from build123d import *

# Parameters (mm, degrees)
SKETCH4_R          = 3
CUT_EXTRUDE1_DEPTH = 1
CUT_EXTRUDE2_START = -3
SKETCH5_R          = 3
CUT_EXTRUDE2_DEPTH = 3
CUT_EXTRUDE3_REACH = 19.282
SKETCH6_R          = 1.143
SKETCH6_R_2        = 1.1938


with BuildPart() as part:
    # Sketch1 → Revolve1 (revolve)
    with BuildSketch(Plane.XY, mode=Mode.PRIVATE) as revolve1_sk:
        Polygon((-12, 0), (-3.75, 0), (-3.75, 1.732400048), (-1.4, 1.732400048), (-1.4, -3.267599952), (-4.45, -3.267599952), (-4.45, -1.700599952), (-12, -1.700599952), align=None)
    revolve(revolve1_sk.sketch.rotate(Axis((0, 0, 0), (0, -1, 0)), 270), axis=Axis((0, 0, 0), (0, -1, 0)))

    # Sketch4 → Cut-Extrude1 (cut)
    with BuildSketch(Plane(origin=(0, 1.732400048, 0), x_dir=(-1, 0, 0), z_dir=(0, 1, 0))):
        with Locations(Location((0, 0, 0), (0, 0, 90))):
            Circle(SKETCH4_R)
    extrude(amount=-CUT_EXTRUDE1_DEPTH, mode=Mode.SUBTRACT)

    # Sketch5 → Cut-Extrude2 (cut)
    with BuildSketch(Plane.XZ.offset(3.267599952).offset(CUT_EXTRUDE2_START)):
        with Locations(Location((0, 0, 0), (0, 0, 90))):
            Circle(SKETCH5_R)
    extrude(amount=CUT_EXTRUDE2_DEPTH, mode=Mode.SUBTRACT)

    # Sketch6 → Cut-Extrude3 (cut, up to next)
    with BuildSketch(Plane(origin=(0, 0, 0), x_dir=(1, 0, 0), z_dir=(0, 1, 0)), mode=Mode.PRIVATE) as cut_extrude3_sk1:
        with Locations(Location((0, 8.3312, 0), (0, 0, 270))):
            Circle(SKETCH6_R)
    cut_extrude3_tool1 = extrude(cut_extrude3_sk1.sketch, amount=-CUT_EXTRUDE3_REACH, mode=Mode.PRIVATE) & part.part
    # Sketch6 → Cut-Extrude3 (cut, up to next)
    with BuildSketch(Plane(origin=(0, 0, 0), x_dir=(1, 0, 0), z_dir=(0, 1, 0)), mode=Mode.PRIVATE) as cut_extrude3_sk2:
        with Locations(Location((-8.3312, 0, 0), (0, 0, 270))):
            Circle(SKETCH6_R)
    cut_extrude3_tool2 = extrude(cut_extrude3_sk2.sketch, amount=-CUT_EXTRUDE3_REACH, mode=Mode.PRIVATE) & part.part
    # Sketch6 → Cut-Extrude3 (cut, up to next)
    with BuildSketch(Plane(origin=(0, 0, 0), x_dir=(1, 0, 0), z_dir=(0, 1, 0)), mode=Mode.PRIVATE) as cut_extrude3_sk3:
        with Locations(Location((0, -8.3312, 0), (0, 0, 270))):
            Circle(SKETCH6_R)
    cut_extrude3_tool3 = extrude(cut_extrude3_sk3.sketch, amount=-CUT_EXTRUDE3_REACH, mode=Mode.PRIVATE) & part.part
    # Sketch6 → Cut-Extrude3 (cut, up to next)
    with BuildSketch(Plane(origin=(0, 0, 0), x_dir=(1, 0, 0), z_dir=(0, 1, 0)), mode=Mode.PRIVATE) as cut_extrude3_sk4:
        with Locations(Location((8.3312, 0, 0), (0, 0, 270))):
            Circle(SKETCH6_R_2)
    cut_extrude3_tool4 = extrude(cut_extrude3_sk4.sketch, amount=-CUT_EXTRUDE3_REACH, mode=Mode.PRIVATE) & part.part
    add(cut_extrude3_tool1.solids().sort_by_distance((0, 0, -8.3312))[0], mode=Mode.SUBTRACT)
    add(cut_extrude3_tool2.solids().sort_by_distance((-8.3312, 0, 0))[0], mode=Mode.SUBTRACT)
    add(cut_extrude3_tool3.solids().sort_by_distance((0, 0, 8.3312))[0], mode=Mode.SUBTRACT)
    add(cut_extrude3_tool4.solids().sort_by_distance((8.3312, 0, 0))[0], mode=Mode.SUBTRACT)


solid = part.part
Build history of the part. All positions in model axes, mm. A direction names the side the tool comes from. Round coordinates to 2 decimals unless told otherwise and drop trailing zeros. Loops run counter-clockwise (first coordinate to the right, second up) from the corner with the lowest first, then second, coordinate; pieces in that order, holes last. Notation, with made-up numbers: (-28.75, 77.25) -> (3.25, 77.25) arc R29 cw to (3.25, 102.25) -> close; hole circle Ø1 at (-17, 40.5). An arc over 180 degrees is marked (long way). One line per item, written item: value. Start each with the question number.
Q1. Cut at C-C on y = 1.05. List the corners of the cut face in (x, z), plus the area to 3 significant figures.
Q2. Drop flat-ended pins along their axis: pin 1 Ø5.5 at (x, z) = (0, 0) entering from +Y; pin 2 Ø3.5 at (x, z) = (-8.33, 0) entering from -Y; pin 3 Ø2 at (y, z) = (0, -8) entering from +X. Give the stop position or say it passes through.
Q3. Cut at D-D on z = -9. List the corners of the cut face in (x, y), plus the area to 3 significant figures.
Q4. Cut at A-A on z = 0. Count the separate pieces of the cut face and the enclosed holes in it, plus the area to 3 significant figures.
Q5. 3-axis set-ups, long thin cutter, end or side, ignore diameter. For faces 4 (the face through (-0.165, 0.878, -3.746)), 5 (the face through (0, -1.701, -5)), 6 (the face through (-3.604, -0.838, 11.446)): which of +Z, -Z, +X, -X, +Y, -Y reach the whole face in a straight line?
Q6. Two-plate mould, pull along Z, no slides. Class faces 1 (the face through (1, -3.268, -3)), 2 (the face through (-0.06, 0.23, -1.4)), 3 (the face through (-3.01, -2.47, -3.28)): released by +Z, released by -Z, zero draft, split by the parting line, or undercut.
Q7. Probe line 1 along Y through (x, z) = (0.25, -9.75); line 2 along X through (y, z) = (0.55, 0); line 3 along Z through (x, y) = (-2.75, -3). List the from-to ranges inside material, lowest first.
Computed:
1. outline: circle Ø7.5 at (0, 0); hole circle Ø6 at (0, 0)
1. area: 15.9 mm²
2. pin 1: y = 0.73
2. pin 2: y = -1.7
2. pin 3: x = 9.75
3. outline: (-7.94, -1.7) -> (-0.93, -1.7) -> (-0.93, 0) -> (-7.94, 0) -> close; (0.93, -1.7) -> (7.94, -1.7) -> (7.94, 0) -> (0.93, 0) -> close
3. area: 23.8 mm²
4. separate pieces: 4
4. enclosed holes: 0
4. area: 33.0 mm²
5. face 4: +Y
5. face 5: -Y
5. face 6: +Y, -Y
6. face 1: zero draft
6. face 2: undercut
6. face 3: split by the parting line
7. line 1: -1.7 to 0
7. line 2: -3.75 to -1.4, 1.4 to 3.75
7. line 3: -3.5 to -1.2, 1.2 to 3.5
